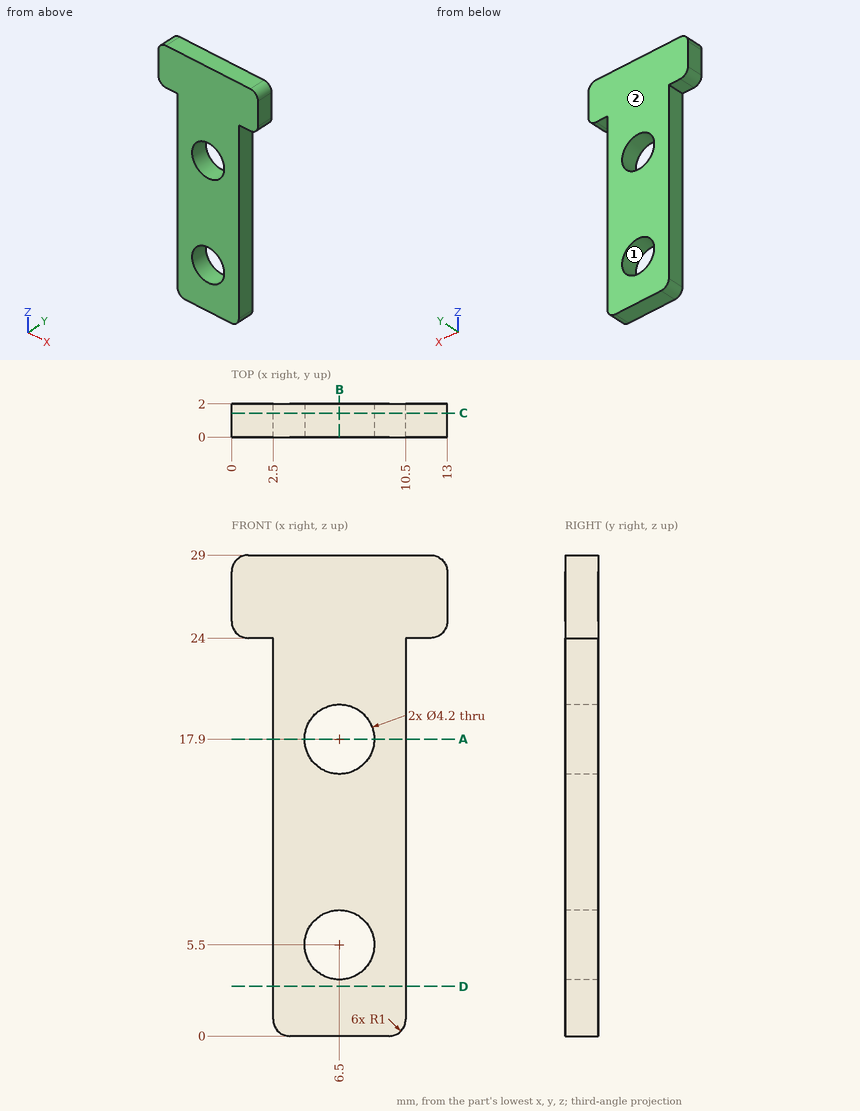
Geometry check sheet. Reference: drawing and pictorial views, mm from the part's lowest x, y, z. Coordinates: 2 decimals unless noted, no trailing zeros. Order: outer loops, then holes, each group sorted by start corner. A loop starts at its lowest first (then second) coordinate and runs counter-clockwise, first axis right, second up. Notation, with made-up numbers: (10, -19) -> (67, -19) arc R10 ccw to (67, -8) -> close; hole circle Ø10 at (84, 15.25). An arc over 180 degrees is marked (long way). Put each result on its own line as item: value. Start each with the question number.
1) Release check for a two-part mould opening along Z. For the marked faces 1 and 2 record: pulls with the +Z half, pulls with the -Z half, needs draft (parallel to the pull), parting line crosses it, or undercut.
2) Cross-section at D-D (z = 3). Enter the section's corners in (x, y).
3) Go/stop test with flat-tipped pins: pin 1 (0.6 mm diameter, centred on y = 1.5, z = 17, fed in from +X); pin 2 (1 mm diameter, centred on y = 1.5, z = 15.5, fed in from -X); pin 3 (4 mm diameter, centred on x = 6.5, z = 5.5, fed in from +Y). Record where each tip stops, or that it passes through.
4) Cross-section at B-B (x = 6.5). Enter the section's corners in (y, z).
5) Material ranges on L1, parallel to X at y = 0.9, z = 17.9; L2, parallel to Z at x = 6, y = 1.6; L3, parallel to Z at x = 11.75, y = 1.65, recorded low to high.
6) Cross-section at C-C (y = 1.45). Enter the section's corners in (x, z).
7) Cross-section at A-A (z = 17.9). Enter the section's corners in (x, y), plus the area to 3 significant figures.
Geometry check:
1. face 1: undercut
1. face 2: needs draft
2. outline: (2.5, 0) -> (10.5, 0) -> (10.5, 2) -> (2.5, 2) -> close
3. pin 1: stops at x = 10.5
3. pin 2: stops at x = 2.5
3. pin 3: passes through
4. outline: (0, 0) -> (2, 0) -> (2, 3.4) -> (0, 3.4) -> close; (0, 7.6) -> (2, 7.6) -> (2, 15.8) -> (0, 15.8) -> close; (0, 20) -> (2, 20) -> (2, 29) -> (0, 29) -> close
5. L1: x = 2.5 to 4.4, 8.6 to 10.5
5. L2: z = 0 to 3.46, 7.54 to 15.86, 19.94 to 29
5. L3: z = 24 to 29
6. outline: (0, 25) arc R1 ccw to (1, 24) -> (2.5, 24) -> (2.5, 1) arc R1 ccw to (3.5, 0) -> (9.5, 0) arc R1 ccw to (10.5, 1) -> (10.5, 24) -> (12, 24) arc R1 ccw to (13, 25) -> (13, 28) arc R1 ccw to (12, 29) -> (1, 29) arc R1 ccw to (0, 28) -> close; hole circle Ø4.2 at (6.5, 5.5); hole circle Ø4.2 at (6.5, 17.9)
7. outline: (2.5, 0) -> (4.4, 0) -> (4.4, 2) -> (2.5, 2) -> close; (8.6, 0) -> (10.5, 0) -> (10.5, 2) -> (8.6, 2) -> close
7. area: 7.60 mm^2
